Geometry: final body of the model. Coordinates: model frame, mm. Face numbers are marked on the shaded views. A direction names the side the tool comes from. Give positions to 0.01 mm unless a question says otherwise; leave off trailing zeros. Write each loop counter-clockwise with the first axis right and the second up, starting at its lowest first coordinate (ties: lowest second). Pieces come first, ordered by that corner, then holes.
Q1. Line query: L1, parallel to X at y = 1.15, z = 3.5; L2, parallel to Z at x = 25.5, y = 5.7; L3, parallel to X at y = 1.9, z = 1.75. Output: solid intervals per line, ascending.
Q2. Cut plane C-C on y = 2.6. Return the cut outline in (x, z).
Q3. Cut plane D-D on z = 8.25. Return the cut outline in (x, y), plus the area to 3 significant figures.
Q4. Cut plane A-A on x = -20.5. Return the cut outline in (y, z).
Q5. Cut plane B-B on z = 4.5. Return the cut outline in (x, y), plus the area to 3 significant figures.
Q6. Draft query along Z for the marked faces 3, 4 and 5. Return one class per face: pulls with the +Z half, pulls with the -Z half, needs draft (parallel to the pull), parting line crosses it, or undercut.
Q7. Reachability of the marked faces 1 and 2 from +Z, -Z, +X, -X, +Y, -Y: full face, straight path, thin tool, end or side. Return the list, or none.
Q8. Pin query (flat end, axial travel): pin 1 (0.5 mm diameter, centred on y = 0.5, z = -3.5, fed in from -X); pin 2 (1.5 mm diameter, centred on y = 3.5, z = 0.5, fed in from +X); pin 3 (3 mm diameter, centred on y = 4.5, z = 10.5, fed in from -X). Return the tip coordinate at first contact, or that it passes through.
```python
from build123d import *

# Parameters (mm, degrees)
ESQUISSE1_W        = 8
ESQUISSE1_H        = 18
BOSS_EXTRU_1_DEPTH = 1
ESQUISSE2_W        = 10
ESQUISSE2_H        = 20
BOSS_EXTRU_2_DEPTH = 5


with BuildPart() as part:
    # Esquisse1 → Boss.-Extru.1 (new body)
    with BuildSketch(Plane(origin=(0, 0, 0), x_dir=(1, 0, 0), z_dir=(0, 1, 0))):
        with BuildLine():
            Line((29.004988077, 12.738826724), (-29.004988077, 12.738826724))
            ThreePointArc((-29.004988077, 12.738826724), (-31.738037586, 6.038637628), (-32.945035587, -1.096153846))
            ThreePointArc((-32.945035587, -1.096153846), (-32.712152787, -5.502218178), (-31.51884357, -9.75))
            ThreePointArc((-31.51884357, -9.75), (-30.739215763, -11.52930192), (-29.859240507, -13.261173276))
            Line((-29.859240507, -13.261173276), (29.859240507, -13.261173276))
            ThreePointArc((29.859240507, -13.261173276), (30.739215763, -11.52930192), (31.51884357, -9.75))
            ThreePointArc((31.51884357, -9.75), (32.712152787, -5.502218178), (32.945035587, -1.096153846))
            ThreePointArc((32.945035587, -1.096153846), (31.738037586, 6.038637628), (29.004988077, 12.738826724))
        make_face()
        with Locations((22.983419658, -0.261173276)):
            Rectangle(ESQUISSE1_W, ESQUISSE1_H, mode=Mode.SUBTRACT)
        with Locations((-22.983419658, -0.261173276)):
            Rectangle(ESQUISSE1_W, ESQUISSE1_H, mode=Mode.SUBTRACT)
        with Locations((0, -0.261173276)):
            Rectangle(ESQUISSE1_W, ESQUISSE1_H, mode=Mode.SUBTRACT)
    extrude(amount=BOSS_EXTRU_1_DEPTH)

    # Esquisse2 → Boss.-Extru.2 (add)
    with BuildSketch(Plane(origin=(0, 1, 0), x_dir=(1, 0, 0), z_dir=(0, 1, 0))):
        with BuildLine():
            Line((-29.004988077, 12.738826724), (29.004988077, 12.738826724))
            ThreePointArc((29.004988077, 12.738826724), (31.738037586, 6.038637628), (32.945035587, -1.096153846))
            ThreePointArc((32.945035587, -1.096153846), (32.712152787, -5.502218178), (31.51884357, -9.75))
            ThreePointArc((31.51884357, -9.75), (30.739215763, -11.52930192), (29.859240507, -13.261173276))
            Line((29.859240507, -13.261173276), (0, -13.261173276))
            Line((0, -13.261173276), (-29.859240507, -13.261173276))
            ThreePointArc((-29.859240507, -13.261173276), (-30.739215763, -11.52930192), (-31.51884357, -9.75))
            ThreePointArc((-31.51884357, -9.75), (-32.712152787, -5.502218178), (-32.945035587, -1.096153846))
            ThreePointArc((-32.945035587, -1.096153846), (-31.738037586, 6.038637628), (-29.004988077, 12.738826724))
        make_face()
        with Locations((-22.983419658, -0.261173276)):
            Rectangle(ESQUISSE2_W, ESQUISSE2_H, mode=Mode.SUBTRACT)
        with Locations((22.983419658, -0.261173276)):
            Rectangle(ESQUISSE2_W, ESQUISSE2_H, mode=Mode.SUBTRACT)
        with Locations((0, -0.261173276)):
            Rectangle(ESQUISSE2_W, ESQUISSE2_H, mode=Mode.SUBTRACT)
    extrude(amount=BOSS_EXTRU_2_DEPTH)


solid = part.part
```
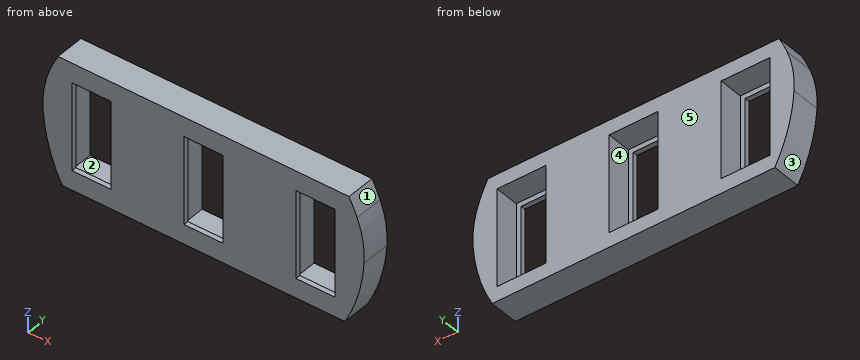
Data:
1. L1: x = -32.94 to -27.98, -17.98 to -5, 5 to 17.98, 27.98 to 32.94
1. L2: z = -12.74 to -9.74, 10.26 to 13.26
1. L3: x = -32.97 to -27.98, -17.98 to -5, 5 to 17.98, 27.98 to 32.97
2. outline: (-32.95, 1.1) arc R33 ccw to (-29, -12.74) - (29, -12.74) arc R33 ccw to (32.95, 1.1) arc R20 ccw to (31.52, 9.75) arc R34 ccw to (29.86, 13.26) - (-29.86, 13.26) arc R34 ccw to (-31.52, 9.75) arc R20 ccw to start; hole (-27.98, -9.74) - (-17.98, -9.74) - (-17.98, 10.26) - (-27.98, 10.26) - close; hole (-5, -9.74) - (5, -9.74) - (5, 10.26) - (-5, 10.26) - close; hole (17.98, -9.74) - (27.98, -9.74) - (27.98, 10.26) - (17.98, 10.26) - close
3. outline: (-32.06, 0) - (-26.98, 0) - (-26.98, 1) - (-27.98, 1) - (-27.98, 6) - (-32.06, 6) - close; (-18.98, 0) - (-4, 0) - (-4, 1) - (-5, 1) - (-5, 6) - (-17.98, 6) - (-17.98, 1) - (-18.98, 1) - close; (4, 0) - (18.98, 0) - (18.98, 1) - (17.98, 1) - (17.98, 6) - (5, 6) - (5, 1) - (4, 1) - close; (26.98, 0) - (32.06, 0) - (32.06, 6) - (27.98, 6) - (27.98, 1) - (26.98, 1) - close
3. area: 211 mm2
4. outline: (0, -12.74) - (6, -12.74) - (6, -9.74) - (1, -9.74) - (1, -8.74) - (0, -8.74) - close; (0, 9.26) - (1, 9.26) - (1, 10.26) - (6, 10.26) - (6, 13.26) - (0, 13.26) - close
5. outline: (-32.85, 0) - (-26.98, 0) - (-26.98, 1) - (-27.98, 1) - (-27.98, 6) - (-32.85, 6) - close; (-18.98, 0) - (-4, 0) - (-4, 1) - (-5, 1) - (-5, 6) - (-17.98, 6) - (-17.98, 1) - (-18.98, 1) - close; (4, 0) - (18.98, 0) - (18.98, 1) - (17.98, 1) - (17.98, 6) - (5, 6) - (5, 1) - (4, 1) - close; (26.98, 0) - (32.85, 0) - (32.85, 6) - (27.98, 6) - (27.98, 1) - (26.98, 1) - close
5. area: 220 mm2
6. face 3: pulls with the -Z half
6. face 4: undercut
6. face 5: needs draft
7. face 1: +Z, +X, +Y, -Y
7. face 2: +Y
8. pin 1: stops at x = -32.4
8. pin 2: stops at x = 32.95
8. pin 3: stops at x = -31.8
